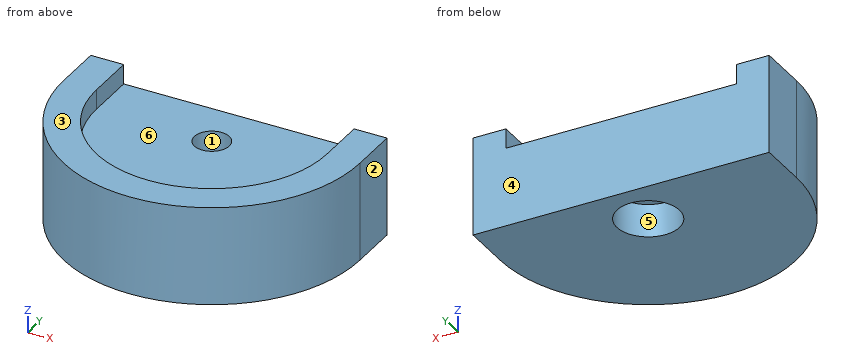
```python
from build123d import *

# Parameters (mm, degrees)
EXTRUDE_1_DEPTH          = 25
CUT_EXTRUDE_1_DEPTH      = 3
CUT_EXTRUDE_2_DEPTH      = 20
CUT_EXTRUDE_2_DEPTH_BACK = 35
SKETCH_3_W               = 45
SKETCH_3_H               = 15
SKETCH_4_R               = 2.65
CUT_EXTRUDE_3_DEPTH      = 35
SKETCH_5_R               = 4.75
CUT_EXTRUDE_4_DEPTH      = 15
SKETCH_6_R               = 24.891831438
CUT_EXTRUDE_5_DEPTH      = 10


with BuildPart() as part:
    # 草图1 → 凸台-拉伸1 (new body)
    with BuildSketch(Plane.XY):
        with BuildLine():
            Line((-22.5, 0), (-22.5, 22.5))
            Line((-22.5, 22.5), (22.5, 22.5))
            Line((22.5, 22.5), (22.5, 0))
            ThreePointArc((22.5, 0), (0, -22.5), (-22.5, 0))
        make_face()
    extrude(amount=EXTRUDE_1_DEPTH)

    # 草图2 → 切除-拉伸1 (cut)
    with BuildSketch(Plane.XY.offset(25)):
        with BuildLine():
            Line((17.5, 22.5), (-17.5, 22.5))
            Line((-17.5, 22.5), (-17.5, 0))
            ThreePointArc((-17.5, 0), (0, 17.5), (17.5, 0))
            Line((17.5, 0), (17.5, 22.5))
        make_face()
        with BuildLine():
            ThreePointArc((17.5, 0), (0, 17.5), (-17.5, 0))
            Line((-17.5, 0), (17.5, 0))
        make_face()
        with BuildLine():
            Line((17.5, 0), (-17.5, 0))
            ThreePointArc((-17.5, 0), (0, -17.5), (17.5, 0))
        make_face()
    extrude(amount=-CUT_EXTRUDE_1_DEPTH, mode=Mode.SUBTRACT)

    # 草图3 → 切除-拉伸2 (cut, two sides: drawn at the far end of the back side and taken through both)
    with BuildSketch(Plane.XY.offset(22).offset(-CUT_EXTRUDE_2_DEPTH_BACK)):
        with Locations((0, 15)):
            Rectangle(SKETCH_3_W, SKETCH_3_H)
    extrude(amount=CUT_EXTRUDE_2_DEPTH + CUT_EXTRUDE_2_DEPTH_BACK, mode=Mode.SUBTRACT)

    # 草图4 → 切除-拉伸3 (cut)
    with BuildSketch(Plane.XY.offset(22)):
        Circle(SKETCH_4_R)
    extrude(amount=-CUT_EXTRUDE_3_DEPTH, mode=Mode.SUBTRACT)

    # 草图5 → 切除-拉伸4 (cut)
    with BuildSketch(Plane(origin=(0, 0, 0), x_dir=(-1, 0, 0), z_dir=(0, 0, -1))):
        Circle(SKETCH_5_R)
    extrude(amount=-CUT_EXTRUDE_4_DEPTH, mode=Mode.SUBTRACT)

    # 草图6 → 切除-拉伸5 (cut)
    with BuildSketch(Plane(origin=(0, 0, 0), x_dir=(-1, 0, 0), z_dir=(0, 0, -1))):
        Circle(SKETCH_6_R)
    extrude(amount=-CUT_EXTRUDE_5_DEPTH, mode=Mode.SUBTRACT)


solid = part.part
```
Input: part model. Units: mm. Frame: model coordinates. Face numbers are marked on the shaded views. A direction names the side the tool comes from. Round coordinates to 2 decimals unless told otherwise and drop trailing zeros. Loops run counter-clockwise (first coordinate to the right, second up) from the corner with the lowest first, then second, coordinate; pieces in that order, holes last. Notation, with made-up numbers: M 80.25,88.5 L 97.25,88.5 A31 ccw 97.25,124.5 Z; hole C 4.25,48.25 d7. An arc over 180 degrees is marked long. Answer in a Markdown table with one row per item. Add a question column.
1. Section C-C (y = -11.75). Output: boundary loops of the cut face in (x, z).
2. Set-up query: the marked faces 4, 5 and 6. Return all of +Z, -Z, +X, -X, +Y, -Y with unobstructed straight access to the full face (end or side cutting, diameter ignored); none if empty.
3. Section B-B (z = 12.5). Output: boundary loops of the cut face in (x, y).
4. Mould query, pull axis X, two halves, no side actions, for the marked faces 1, 2 and 3. Classes: released by +X, released by -X, zero draft, split by the parting line, or undercut.
5. Section D-D (z = 22.75). Output: boundary loops of the cut face in (x, y), and give its area (3 significant figures).
6. Ray query, probe 1 along Y at (x, z) = (0, 17.5); probe 2 along Z at (x, y) = (-6, -13); probe 3 along X at (y, z) = (-3.25, 22.75). Return the intervals inside material, ascending.
7. Section A-A (x = 0). Output: boundary loops of the cut face in (y, z), and give its area (3 significant figures).
8. Contact query for flat-ended pins moving along their axis: pin 1 (6 mm diameter, centred on y = -9.5, z = 23.5, fed in from -X); pin 2 (12.5 mm diameter, centred on x = 2, y = -9.5, fed in from +Z); pin 3 (7.5 mm diameter, centred on x = 0.5, y = 0.5, fed in from -Z). Output: stop coordinate, or through.
Values follow:
| question | item | result |
|---|---|---|
| 1 | outline | M -19.19,10 L 19.19,10 L 19.19,25 L 12.97,25 L 12.97,22 L -12.97,22 L -12.97,25 L -19.19,25 Z |
| 2 | face 4 | +Z, -Z, +X, -X, +Y |
| 2 | face 5 | -Z |
| 2 | face 6 | +Z, +Y |
| 3 | outline | M -22.5,0 A22.5 ccw 22.5,0 L 22.5,7.5 L -22.5,7.5 Z; hole C 0,0 d9.5 |
| 4 | face 1 | undercut |
| 4 | face 2 | released by +X |
| 4 | face 3 | zero draft |
| 5 | outline | M -22.5,0 A22.5 ccw 22.5,0 L 22.5,7.5 L 17.5,7.5 L 17.5,0 A17.5 cw -17.5,0 L -17.5,7.5 L -22.5,7.5 Z |
| 5 | area | 389 mm^2 |
| 6 | probe 1 | -22.5 to -2.65, 2.65 to 7.5 |
| 6 | probe 2 | 10 to 22 |
| 6 | probe 3 | -22.26 to -17.2, 17.2 to 22.26 |
| 7 | outline | M -22.5,10 L -4.75,10 L -4.75,15 L -2.65,15 L -2.65,22 L -17.5,22 L -17.5,25 L -22.5,25 Z; M 2.65,15 L 4.75,15 L 4.75,10 L 7.5,10 L 7.5,22 L 2.65,22 Z |
| 7 | area | 290 mm^2 |
| 8 | pin 1 | x = -21.54 |
| 8 | pin 2 | z = 22 |
| 8 | pin 3 | z = 15 |
